Autodesk Inventor part; units mm, degrees
ref_plane "YZ Plane" through (0, 0, 0) normal (1, 0, 0) x (0, 1, 0)
ref_plane "XZ Plane" through (0, 0, 0) normal (0, 1, 0) x (-1, 0, 0)
ref_plane "XY Plane" through (0, 0, 0) normal (0, 0, 1) x (1, 0, 0)
sketch "Sketch1" plane through (0, 0, 0) normal (0, 0, 1) x (1, 0, 0)
  line L0 (0, 0) -> (34, 0)
  line L1 (34, 0) -> (34, 18)
  line L2 (34, 18) -> (0, 18)
  line L3 (0, 18) -> (0, 0)
  line L4 (-6, 16) -> (0, 16)
  line L5 (0, 16) -> (0, 6)
  line L6 (0, 6) -> (-6, 6)
  line L7 (-6, 6) -> (-6, 16)
  line L8 (-6, 16) -> (0, 6) construction
  line L9 (0, 16) -> (-6, 6) construction
  line L10 (38, 16) -> (34, 16)
  line L11 (34, 16) -> (34, 6)
  line L12 (34, 6) -> (38, 6)
  line L13 (38, 6) -> (38, 16)
  line L14 (38, 16) -> (34, 6) construction
  line L15 (34, 16) -> (38, 6) construction
  point P0 (-3, 11)
  point P1 (36, 11)
  point P2 (0, 16)
  dimension "d0" = 34
  dimension "d2" = 4
  dimension "d3" = 6
  dimension "d4" = 10
  dimension "d5" = 10
  dimension "d8" = 6
  dimension "d9" = 2
extrude "Extrusion1" add sketch "Sketch1" along normal blind 3
properties part number "Frontrail"
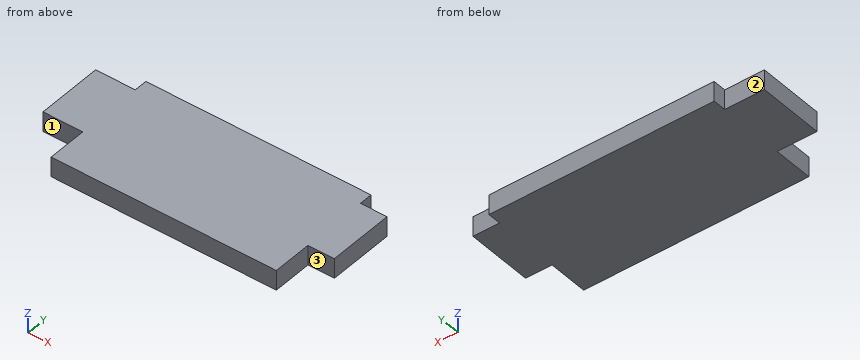
Design review of the part built by this model. Coordinates are the model's own, in mm. Face numbers are marked on the shaded views. A direction names the side the tool comes from. Coordinates: 2 decimals unless noted, no trailing zeros. Order: outer loops, then holes, each group sorted by start corner. A loop starts at its lowest first (then second) coordinate and runs counter-clockwise, first axis right, second up.
1) For the marked faces 1, 2 and 3, list the 3-axis set-ups (+Z, -Z, +X, -X, +Y, -Y) from which the entire face can be reached by the end or side of a thin tool; tool diameter is ignored.
2) Clearance check with flat-ended pins moving along their axes: pin 1 (1.6 mm diameter, centred on y = 17, z = 2, fed in from +X); pin 2 (1.5 mm diameter, centred on x = 8.5, y = 9.5, fed in from -Z); pin 3 (0.9 mm diameter, centred on y = 3, z = 1.5, fed in from -X). State where each tip first meets the part, or that it passes through.
3) Take a section at B-B, the plane x = -1. Give the boundary of the cut face in (y, z), and give its area (3 significant figures).
4) Wall thickness on line 1 along X through (y, z) = (4, 2.15); line 2 along Y through (x, z) = (-3, 2.6): over which ranges is each line inside the solid? List them lowest first.
5) Take a section at A-A, the plane z = 1.25. Give the boundary of the cut face in (x, y), and give its area (3 significant figures).
6) Take a section at C-C, the plane y = 4.5. Give the boundary of the cut face in (x, z).
Returned:
1. face 1: +Z, -Z, -X, -Y
1. face 2: +Z, -Z, -X, +Y
1. face 3: +Z, -Z, +X, -Y
2. pin 1: stops at x = 34
2. pin 2: stops at z = 0
2. pin 3: stops at x = 0
3. outline: (6, 0) - (16, 0) - (16, 3) - (6, 3) - close
3. area: 30.0 mm2
4. line 1: x = 0 to 34
4. line 2: y = 6 to 16
5. outline: (-6, 6) - (0, 6) - (0, 0) - (34, 0) - (34, 6) - (38, 6) - (38, 16) - (34, 16) - (34, 18) - (0, 18) - (0, 16) - (-6, 16) - close
5. area: 712 mm2
6. outline: (0, 0) - (34, 0) - (34, 3) - (0, 3) - close
